```python
from build123d import *

# Parameters (mm, degrees)
F0_W         = 45
F0_H         = 45
F1_DEPTH     = 2
F3_DEPTH     = 45
F5_DEPTH     = 50
F7_DEPTH     = 52.4
F9_DEPTH     = 6.25
F10_T1_DEPTH = 62.3121019707
F11_T1_DEPTH = 49.4942070429


# Not quite as in the source:
# - a fillet or chamfer that OpenCascade refuses, or shapes differently, is made with other operations: its cross-section is extruded or revolved along the edge and cut away or added


with BuildPart() as f1:
    # F0 (on Top) → F1 (new body)
    with BuildSketch(Plane.XY):
        with Locations((-22.5, 22.5)):
            Rectangle(F0_W, F0_H)
    extrude(amount=F1_DEPTH)

    # F2 (on Front) → F3 (join)
    with BuildSketch(Plane.XZ):
        with BuildLine():
            Line((-45, 0), (0, 0))
            Line((0, 0), (-3, 52))
            Line((-3, 52), (-32.9244207251, 42.7682981249))
            ThreePointArc((-32.9244207251, 42.7682981249), (-34.5043559539, 20.1254790506), (-45, 0))
        make_face()
    extrude(amount=-F3_DEPTH)

    # F4 (on Right) → F5 (cut)
    with BuildSketch(Plane.YZ):
        Polygon((0, 0), (12.5, 59.1310895979), (0, 59.1310895979), align=None)
        Polygon((45, 0), (45, 59.1310895979), (32.5, 59.1310895979), align=None)
    extrude(amount=-F5_DEPTH, mode=Mode.SUBTRACT)

    # F6 (on Right) → F7 (cut)
    with BuildSketch(Plane.YZ):
        Polygon((37.7679802477, 54.4090420008), (10.9807690606, 52.094515413), (37.7679802477, 42.2525405884), align=None)
    extrude(amount=-F7_DEPTH, mode=Mode.SUBTRACT)

    # F8 (on face) → F9 (cut)
    with BuildSketch(Plane(origin=(0, 18.1697536282, 49.4531876304), x_dir=(1, 0, 0), z_dir=(0, 0.3448722583, 0.9386496287))):
        Polygon((-14.9190827221, 18.9156103945), (-13.4748989156, 42.5651032579), (-19.9628132083, 42.9612952953), (-21.4311909427, 18.9156103945), align=None)
        Polygon((-15.8245932316, 4.0872594346), (-14.9190827221, 18.9156103945), (-21.4311909427, 18.9156103945), (-21.9993973802, 9.6108432114), align=None)
        Polygon((-17.0844251269, -16.5433453977), (-15.8245932316, 4.0872594346), (-21.9993973802, 9.6108432114), (-23.5723394196, -16.1471533603), align=None)
    extrude(amount=-F9_DEPTH, mode=Mode.SUBTRACT)

    # F10: fillet of radius 5 on 1 edges, made by hand

    # F10_s2 → F10_t1 (cut)
    with BuildSketch(Plane.XZ.offset(-53.6560509853)):
        with BuildLine():
            ThreePointArc((-45, -1.6315361684), (-44.5926166392, 0.3452977662), (-43.436851038, 2))
            Line((-43.436851038, 2), (-45, 2))
            Line((-45, 2), (-45, -1.6315361684))
        make_face()
    extrude(amount=F10_T1_DEPTH, mode=Mode.SUBTRACT)

    # F11: fillet of radius 5 on 1 edges, made by hand

    # F11_s2 → F11_t1 (cut)
    with BuildSketch(Plane.XZ.offset(-47.2471035215)):
        with BuildLine():
            ThreePointArc((0, 0.9320428172), (-0.0289298475, 1.4691289727), (-0.1153846154, 2))
            Line((-0.1153846154, 2), (0, 2))
            Line((0, 2), (0, 0.9320428172))
        make_face()
    extrude(amount=F11_T1_DEPTH, mode=Mode.SUBTRACT)


solid = f1.part
```
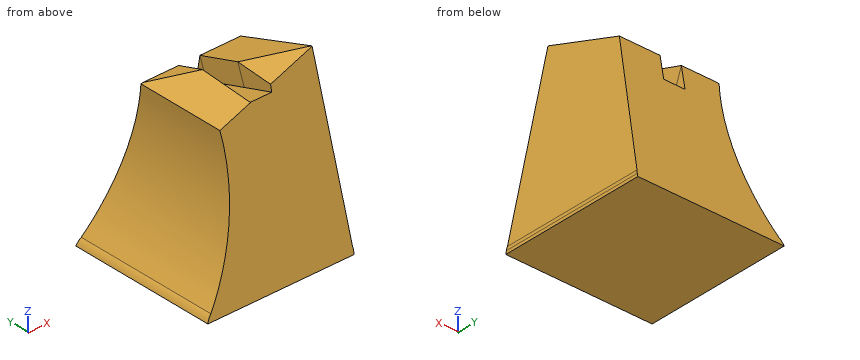
Geometry check sheet. Reference: the model listing, model coordinates, mm. Give positions to 0.01 mm unless a question says otherwise; leave off trailing zeros. Loops run counter-clockwise (first coordinate to the right, second up) from the corner with the lowest first, then second, coordinate; pieces in that order, holes last. Notation, with made-up numbers: (80, 33.5) - (111, 33.5) arc R23 ccw to (111, 62.5) - close; hole circle Ø4 at (8.5, -37). An arc over 180 degrees is marked (long way). Use CSV: the item, a comma, the result in double quotes. Start each with the question number.
Q1. Section check C-C, the plane z = 11.5. Record the cut outline in (x, y).
Q2. Section check A-A, the plane y = 8. Record the cut outline in (x, z), and give its area (3 significant figures).
Q3. Section check B-B, the plane x = -19. Record the cut outline in (y, z), and give its area (3 significant figures).
Q4. Go/stop test with flat-tipped pins: pin 1 Ø5 at (y, z) = (13, 22.5) entering from -X; pin 2 Ø1.5 at (y, z) = (30, 44) entering from +X; pin 3 Ø10 at (x, z) = (-32.5, 32.5) entering from -Y. Record where each tip stops, or that it passes through.
Q5. Scan lines: probe 1 along X at (y, z) = (36, 39); probe 2 along Z at (x, y) = (-15, 25); probe 3 along X at (y, z) = (11, 41). Record each from-to range of solid material in increasing order. Write a range as from..to.
Q6. Section check D-D, the plane y = 16. Record the cut outline in (x, z), and give its area (3 significant figures).
Findings below:
1,outline,"(-37.73, 2.43) - (-0.66, 2.43) - (-0.66, 42.57) - (-37.73, 42.57) - close"
2,outline,"(-44.73, 0) - (0, 0) - (0, 0.93) arc R5 ccw to (-0.12, 2) - (-2.18, 37.84) - (-32.47, 37.84) arc R55.61 cw to (-43.44, 2) arc R5 ccw to start"
2,area,"1,330 mm^2"
3,outline,"(0, 0) - (45, 0) - (37.45, 35.71) - (9.7, 45.91) - close"
3,area,"1,490 mm^2"
4,pin 1,"stops at x = -34.54"
4,pin 2,"stops at x = -2.5"
4,pin 3,"stops at y = 5.81"
5,probe 1,"x = -32.54..-21.34, -14.83..-2.25"
5,probe 2,"z = 0..46.94"
5,probe 3,"x = -32.71..-2.37"
6,outline,"(-44.73, 0) - (0, 0) - (0, 0.93) arc R5 ccw to (-0.12, 2) - (-2.9, 50.25) - (-8.67, 50.25) - (-16.17, 47.94) - (-16.08, 43.59) - (-22.59, 43.59) - (-22.64, 45.94) - (-32.92, 42.77) arc R55.61 cw to (-43.44, 2) arc R5 ccw to start"
6,area,"1,590 mm^2"
